Model file for the job. Use its own axes, mm. A direction names the side the tool comes from. Give positions to 0.01 mm unless a question says otherwise; leave off trailing zeros. Write each loop counter-clockwise with the first axis right and the second up, starting at its lowest first coordinate (ties: lowest second). Pieces come first, ordered by that corner, then holes.
```python
from build123d import *

# Parameters (mm, degrees)
SKETCH1_R           = 1.5
BOSS_EXTRUDE1_DEPTH = 12
SKETCH2_R           = 3
BOSS_EXTRUDE2_DEPTH = 2
CUT_EXTRUDE1_DEPTH  = 1.5
FILLET1_R           = 2


with BuildPart() as part:
    # Sketch1 → Boss-Extrude1 (new body)
    with BuildSketch(Plane.XY):
        Circle(SKETCH1_R)
    extrude(amount=BOSS_EXTRUDE1_DEPTH)

    # Sketch2 → Boss-Extrude2 (add)
    with BuildSketch(Plane.XY.offset(12)):
        Circle(SKETCH2_R)
    extrude(amount=BOSS_EXTRUDE2_DEPTH)

    # Sketch3 → Cut-Extrude1 (cut)
    with BuildSketch(Plane.XY.offset(14)):
        Polygon((-1.732050808, 0), (-0.866025404, -1.5), (0.866025404, -1.5), (1.732050808, 0), (0.866025404, 1.5), (-0.866025404, 1.5), align=None)
    extrude(amount=-CUT_EXTRUDE1_DEPTH, mode=Mode.SUBTRACT)

    # Fillet1
    # the kernel refuses this fillet: 2 mm, written as the material it takes off along each edge
    with BuildSketch(Plane(origin=(0, 0, 14), x_dir=(1, 0, 0), z_dir=(0, -1, 0))) as fillet1_piece_1:
        with BuildLine():
            CenterArc((3 - FILLET1_R, -FILLET1_R), FILLET1_R, 0, 90)
            Line((3 - FILLET1_R, 0), (3, 0))
            Line((3, 0), (3, -FILLET1_R))
        make_face()
    revolve(axis=Axis((0, 0, 14), (0, 0, 1)), mode=Mode.SUBTRACT)


solid = part.part
```
1. Which spindle directions (+Z, -Z, +X, -X, +Y, -Y) get a long thin tool onto all of the face, cutting with end or side? Do faces 4 (the flat face through (1.3, -1.3, 12)), 5 (the flat face through (1.305, 0.74, 13.228)). Say none if no direction does.
Calculated:
face 4: -Z
face 5: +Z
2. Pin check, flat tips, straight feed: P1, Ø2, axis at y = -1.5, z = 7, coming from the -X side; P2, Ø1, axis at y = 1.5, z = 9, coming from the -X side; P3, Ø1.6, axis at x = 0.5, z = 13, coming from the -Y side. Stop position of each tip, or through.
Calculated:
P1: stops at x = -1.41
P2: stops at x = -1.12
P3: stops at y = -2.98
3. Pull direction X, two halves, no side cores. Call faces 1 (the flat face through (0, 0, 0)), 2 (the cylindrical face through (-1.5, 0.07, 5.92)), 3 (the flat face through (-1.293, 0.76, 13.228)): +X half, -X half, draft (parallel to the pull), parting line (faces both ways), or undercut.
Calculated:
face 1: draft
face 2: parting line
face 3: undercut
4. Slice it at A-A, the plane z = 9. Write the cut outline in (x, y).
Calculated:
outline: circle Ø3 at (0, 0)
5. Probe probe 1 along Y at (x, z) = (0, 10); probe 2 along X at (y, z) = (-0.25, 8.25); probe 3 along Z at (x, y) = (-1.25, 2). List the from-to ranges inside material, lowest first.
Calculated:
probe 1: y = -1.5 to 1.5
probe 2: x = -1.48 to 1.48
probe 3: z = 12 to 13.47
